Check sheet for the drawn part. Datum: minimum x, y, z corner. Units: mm. Give positions to 0.01 mm unless a question says otherwise; leave off trailing zeros. Order: outer loops, then holes, each group sorted by start corner. A loop starts at its lowest first (then second) coordinate and runs counter-clockwise, first axis right, second up.
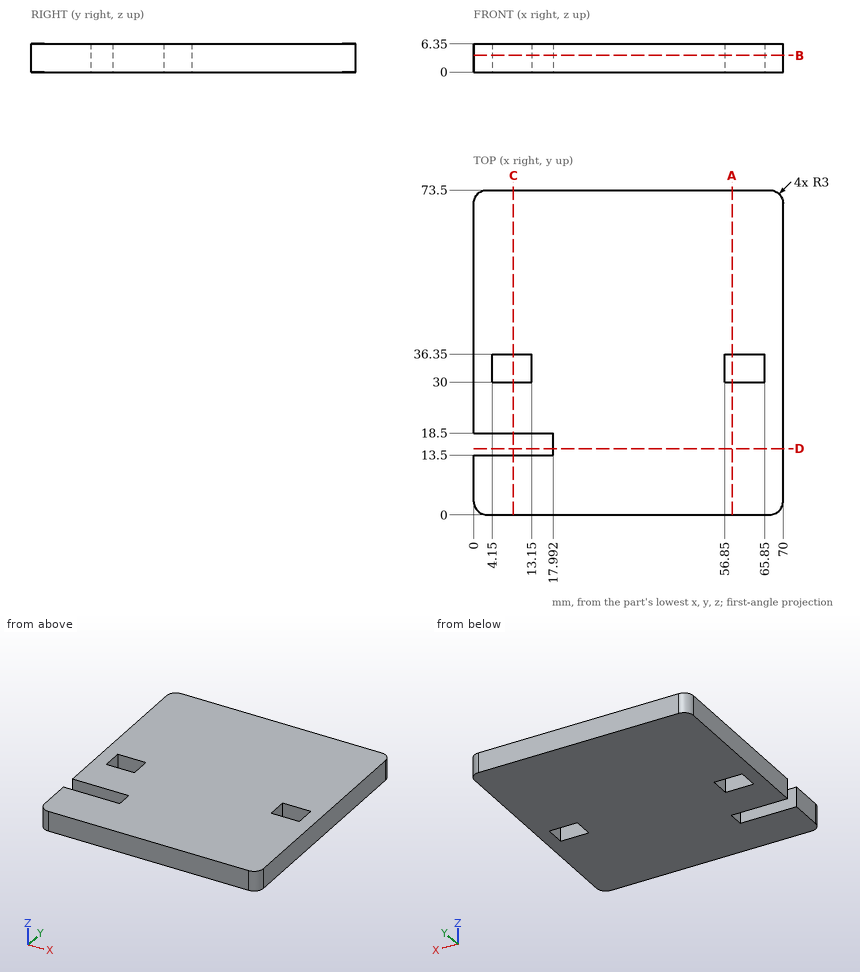
(1) Section check D-D, the plane y = 15. Enter the section's corners in (x, z), then the cut area to 3 significant figures.
Solved:
outline: (17.99, 0) - (70, 0) - (70, 6.35) - (17.99, 6.35) - close
area: 330 mm2
(2) Section check A-A, the plane x = 58.5. Enter the section's corners in (y, z), then the cut area to 3 significant figures.
Solved:
outline: (0, 0) - (30, 0) - (30, 6.35) - (0, 6.35) - close; (36.35, 0) - (73.5, 0) - (73.5, 6.35) - (36.35, 6.35) - close
area: 426 mm2
(3) Section check C-C, the plane x = 9. Enter the section's corners in (y, z), then the cut area to 3 significant figures.
Solved:
outline: (0, 0) - (13.5, 0) - (13.5, 6.35) - (0, 6.35) - close; (18.5, 0) - (30, 0) - (30, 6.35) - (18.5, 6.35) - close; (36.35, 0) - (73.5, 0) - (73.5, 6.35) - (36.35, 6.35) - close
area: 395 mm2
(4) Section check B-B, the plane z = 3.75. Enter the section's corners in (x, y), then the cut area to 3 significant figures.
Solved:
outline: (0, 3) arc R3 ccw to (3, 0) - (67, 0) arc R3 ccw to (70, 3) - (70, 70.5) arc R3 ccw to (67, 73.5) - (3, 73.5) arc R3 ccw to (0, 70.5) - (0, 18.5) - (17.99, 18.5) - (17.99, 13.5) - (0, 13.5) - close; hole (4.15, 30) - (13.15, 30) - (13.15, 36.35) - (4.15, 36.35) - close; hole (56.85, 30) - (65.85, 30) - (65.85, 36.35) - (56.85, 36.35) - close
area: 4,930 mm2
(5) Scan lines: line 1 (Y direction, x = 12, z = 1.75); line 2 (Y direction, x = 58, z = 1.75); line 3 (X direction, y = 33.5, z = 3). Record each from-to range of solid material in increasing order.
Solved:
line 1: y = 0 to 13.5, 18.5 to 30, 36.35 to 73.5
line 2: y = 0 to 30, 36.35 to 73.5
line 3: x = 0 to 4.15, 13.15 to 56.85, 65.85 to 70
(6) Go/stop test with a flat-tipped pin: pin 1 (3 mm diameter, centred on x = 10, z = 5, fed in from -Y). Record where the tip stops, or that it passes through.
Solved:
pin 1: stops at y = 0
